```python
from build123d import *
from build123d.topology import SkipClean

# Parameters (mm, degrees)
SKETCH_1_W           = 51
SKETCH_1_H           = 30
EXTRUDE_5_DEPTH      = 7.5
SKETCH_4_W           = 31
SKETCH_4_H           = 30
EXTRUDE_6_DEPTH      = 20
SKETCH_6_W           = 5.5
SKETCH_6_H           = 10
EXTRUDE_9_DEPTH      = 3
SKETCH_10_W          = 5.5
SKETCH_10_H          = 10
EXTRUDE_10_DEPTH     = 3
SKETCH_13_R          = 10.95
CUT_EXTRUDE_1_DEPTH  = 3.55
CUT_EXTRUDE_2_DEPTH  = 10.3
CUT_EXTRUDE_3_DEPTH  = 33.666075675
CUT_EXTRUDE_5_DEPTH  = 41.391830857
CUT_EXTRUDE_7_DEPTH  = 57.797887285
EXTRUDE_12_DEPTH     = 31
CUT_EXTRUDE_13_DEPTH = 57.79788732
EXTRUDE_14_DEPTH     = 7.5
CUT_EXTRUDE_14_DEPTH = 41.391830988


with BuildPart() as part:
    # Эскиз1 → Бобышка-Вытянуть5 (new body)
    with BuildSketch(Plane.XY):
        Rectangle(SKETCH_1_W, SKETCH_1_H)
    extrude(amount=EXTRUDE_5_DEPTH)

    # Эскиз4 → Бобышка-Вытянуть6 (add)
    with BuildSketch(Plane(origin=(0, 0, 0), x_dir=(-1, 0, 0), z_dir=(0, 0, -1))):
        with Locations((10, 0)):
            Rectangle(SKETCH_4_W, SKETCH_4_H)
    extrude(amount=EXTRUDE_6_DEPTH)

    # Эскиз6 → Бобышка-Вытянуть9 (add)
    with BuildSketch(Plane(origin=(0, 0, 0), x_dir=(-1, 0, 0), z_dir=(0, 0, -1))):
        with Locations((-15.5, 10)):
            Rectangle(SKETCH_6_W, SKETCH_6_H)
        with Locations((-15.5, -10)):
            Rectangle(SKETCH_6_W, SKETCH_6_H)
    extrude(amount=EXTRUDE_9_DEPTH)

    # Эскиз10 → Бобышка-Вытянуть10 (add)
    with BuildSketch(Plane(origin=(5.5, 0, 0), x_dir=(0, 0, -1), z_dir=(1, 0, 0))):
        with Locations((10, 10)):
            Rectangle(SKETCH_10_W, SKETCH_10_H)
        with Locations((10, -10)):
            Rectangle(SKETCH_10_W, SKETCH_10_H)
    extrude(amount=EXTRUDE_10_DEPTH)

    # Эскиз13 → Вырез-Вытянуть1 (cut)
    with BuildSketch(Plane.XY.offset(7.5)):
        with Locations((-10, 0)):
            Circle(SKETCH_13_R)
    extrude(amount=-CUT_EXTRUDE_1_DEPTH, mode=Mode.SUBTRACT)

    # Эскиз14 → Вырез-Вытянуть2 (cut)
    with BuildSketch(Plane.XY.offset(3.95)):
        with BuildLine():
            ThreePointArc((-4.91, 0), (-6.400826484, 3.599173516), (-10, 5.09))
            Line((-10, 5.09), (-10, -5.09))
            ThreePointArc((-10, -5.09), (-6.400826484, -3.599173516), (-4.91, 0))
        make_face()
        with BuildLine():
            Line((-10, -5.09), (-10, 5.09))
            ThreePointArc((-10, 5.09), (-15.09, 0), (-10, -5.09))
        make_face()
    extrude(amount=-CUT_EXTRUDE_2_DEPTH, mode=Mode.SUBTRACT)

    # Эскиз15 → Вырез-Вытянуть3 (cut, through all)
    with BuildSketch(Plane.XY.offset(-6.35)):
        with BuildLine():
            ThreePointArc((-5.7, 0), (-6.959440841, 3.040559159), (-10, 4.3))
            Line((-10, 4.3), (-10, -4.3))
            ThreePointArc((-10, -4.3), (-6.959440841, -3.040559159), (-5.7, 0))
        make_face()
        with BuildLine():
            Line((-10, -4.3), (-10, 4.3))
            ThreePointArc((-10, 4.3), (-14.3, 0), (-10, -4.3))
        make_face()
    extrude(amount=-CUT_EXTRUDE_3_DEPTH, mode=Mode.SUBTRACT)

    # Эскиз16 → Вырез-Вытянуть5 (cut, through all)
    with BuildSketch(Plane.XY.offset(7.5)):
        with BuildLine():
            ThreePointArc((18.3, 0), (17.479898987, 1.979898987), (15.5, 2.8))
            Line((15.5, 2.8), (15.5, -2.8))
            ThreePointArc((15.5, -2.8), (17.479898987, -1.979898987), (18.3, 0))
        make_face()
        with BuildLine():
            Line((15.5, -2.8), (15.5, 2.8))
            ThreePointArc((15.5, 2.8), (12.7, 0), (15.5, -2.8))
        make_face()
    extrude(amount=-CUT_EXTRUDE_5_DEPTH, mode=Mode.SUBTRACT)

    # Эскиз17 → Вырез-Вытянуть7 (cut, through all)
    with SkipClean():  # the faces are left unmerged after this step: merging them gives an invalid solid
        with BuildSketch(Plane.ZY.offset(25.5)):
            with BuildLine():
                ThreePointArc((-12.6, 0), (-10, -2.6), (-7.4, 0))
                Line((-7.4, 0), (-12.6, 0))
            make_face()
            with BuildLine():
                Line((-12.6, 0), (-7.4, 0))
                ThreePointArc((-7.4, 0), (-10, 2.6), (-12.6, 0))
            make_face()
        extrude(amount=-CUT_EXTRUDE_7_DEPTH, mode=Mode.SUBTRACT)

    # Эскиз23 → Бобышка-Вытянуть12 (add)
    with SkipClean():  # the faces are left unmerged after this step: merging them gives an invalid solid
        with BuildSketch(Plane.ZY.offset(25.5)):
            with BuildLine():
                ThreePointArc((-12.6, 0), (-10, -2.6), (-7.4, 0))
                Line((-7.4, 0), (-12.6, 0))
            make_face()
            with BuildLine():
                Line((-12.6, 0), (-7.4, 0))
                ThreePointArc((-7.4, 0), (-10, 2.6), (-12.6, 0))
            make_face()
        extrude(amount=-EXTRUDE_12_DEPTH)

    # Эскиз24 → Вырез-Вытянуть13 (cut, through all)
    with BuildSketch(Plane.ZY.offset(25.5)):
        with BuildLine():
            ThreePointArc((-7.15, 0), (-10, 2.85), (-12.85, 0))
            Line((-12.85, 0), (-7.15, 0))
        make_face()
        with BuildLine():
            Line((-7.15, 0), (-12.85, 0))
            ThreePointArc((-12.85, 0), (-10, -2.85), (-7.15, 0))
        make_face()
    extrude(amount=-CUT_EXTRUDE_13_DEPTH, mode=Mode.SUBTRACT)

    # Эскиз27 → Бобышка-Вытянуть14 (add)
    with BuildSketch(Plane.XY.offset(7.5)):
        with BuildLine():
            ThreePointArc((15.5, 2.8), (12.7, 0), (15.5, -2.8))
            Line((15.5, -2.8), (15.5, 2.8))
        make_face()
        with BuildLine():
            Line((15.5, 2.8), (15.5, -2.8))
            ThreePointArc((15.5, -2.8), (17.479898987, -1.979898987), (18.3, 0))
            ThreePointArc((18.3, 0), (17.479898987, 1.979898987), (15.5, 2.8))
        make_face()
    extrude(amount=-EXTRUDE_14_DEPTH)

    # Эскиз28 → Вырез-Вытянуть14 (cut, through all)
    with BuildSketch(Plane.XY.offset(7.5)):
        with BuildLine():
            ThreePointArc((15.5, 2.85), (12.65, 0), (15.5, -2.85))
            Line((15.5, -2.85), (15.5, 2.85))
        make_face()
        with BuildLine():
            Line((15.5, 2.85), (15.5, -2.85))
            ThreePointArc((15.5, -2.85), (17.515254326, -2.015254326), (18.35, 0))
            ThreePointArc((18.35, 0), (17.515254326, 2.015254326), (15.5, 2.85))
        make_face()
    extrude(amount=-CUT_EXTRUDE_14_DEPTH, mode=Mode.SUBTRACT)


solid = part.part
```
Here's how the part is built. I have some questions about the finished solid (model axes, mm). A direction names the side the tool comes from. Coordinates: 2 decimals unless noted, no trailing zeros. Order: outer loops, then holes, each group sorted by start corner. A loop starts at its lowest first (then second) coordinate and runs counter-clockwise, first axis right, second up. Notation, with made-up numbers: (-26.5, 27) -> (25.5, 27) arc R6 ccw to (25.5, 34) -> close; hole circle Ø9 at (-36, -21.75). An arc over 180 degrees is marked (long way). Return JSON: item names as keys, results as strings.
1) If we section it at D-D on y = -12.5: List the corners of the cut face in (x, z) for me, plus the area to 3 significant figures.
Conclusion:
{"outline": "(-25.5, -20) -> (5.5, -20) -> (5.5, -12.75) -> (8.5, -12.75) -> (8.5, -7.25) -> (5.5, -7.25) -> (5.5, 0) -> (12.75, 0) -> (12.75, -3) -> (18.25, -3) -> (18.25, 0) -> (25.5, 0) -> (25.5, 7.5) -> (-25.5, 7.5) -> close", "area": "1,040 mm²"}
2) Thinking about a two-plate mould opening in X: for faces 1 (the flat face through (12.75, -10, -1)), 2 (the flat face through (7, 10, -12.75)), 3 (the flat face through (8.5, 10, -10)), which applies, +X half, -X half, draft (parallel to the pull), parting line (faces both ways), or undercut?
Conclusion:
{"face 1": "undercut", "face 2": "draft", "face 3": "+X half"}
3) If we section it at B-B on x = 6.5: List the corners of the cut face in (y, z) for me.
Conclusion:
{"outline": "(-15, -12.75) -> (-5, -12.75) -> (-5, -7.25) -> (-15, -7.25) -> close; (-15, 0) -> (15, 0) -> (15, 7.5) -> (-15, 7.5) -> close; (5, -12.75) -> (15, -12.75) -> (15, -7.25) -> (5, -7.25) -> close"}
4) I'm going to push flat-ended pins straight in: P1, Ø1.6, axis at y = 11.5, z = -10.5, coming from the +X side; P2, Ø17.5, axis at x = -10, y = 0, coming from the +Z side; P3, Ø4.5, axis at x = 16, y = 11, coming from the -Z side; P4, Ø1, axis at x = 8, z = -14.5, coming from the +Y side. Where does each tip first touch, or does it pass through?
Conclusion:
{"P1": "stops at x = 8.5", "P2": "stops at z = 3.95", "P3": "stops at z = -3", "P4": "passes through"}
5) If we section it at C-C on y = -2.25: State how many separate pieces and enclosed holes the cut face has, plus the area to 3 significant figures.
Conclusion:
{"separate pieces": "5", "enclosed holes": "0", "area": "623 mm²"}
6) If we section it at A-A on z = -10: List the corners of the cut face in (x, y) for me, plus the area to 3 significant figures.
Conclusion:
{"outline": "(-25.5, -15) -> (8.5, -15) -> (8.5, -5) -> (5.5, -5) -> (5.5, -2.85) -> (-6.78, -2.85) arc R4.3 cw to (-13.22, -2.85) -> (-25.5, -2.85) -> close; (-25.5, 2.85) -> (-13.22, 2.85) arc R4.3 cw to (-6.78, 2.85) -> (5.5, 2.85) -> (5.5, 5) -> (8.5, 5) -> (8.5, 15) -> (-25.5, 15) -> close", "area": "800 mm²"}
7) If I drill on probe 1 along Y at (x, z) = (0.25, -10); probe 2 along Z at (x, y) = (2.5, 0); probe 3 along Y at (x, z) = (-10, 4.7), over which ranges is the centre line in solid material (lowest first)?
Conclusion:
{"probe 1": "y = -15 to -2.85, 2.85 to 15", "probe 2": "z = -20 to -12.85, -7.15 to 7.5", "probe 3": "y = -15 to -10.95, 10.95 to 15"}
8) On a 3-axis mill with a long thin cutter (end or side, diameter ignored), from which of +Z, -Z, +X, -X, +Y, -Y can I reach the whole of each face in a straight line? I mean faces 4 (the flat face through (8.5, -10, -10)), 5 (the flat face through (7, 5, -10)), 6 (the flat face through (12.75, 10, -1)), 7 (the flat face through (7, -10, -7.25)). Say none if no direction works.
Conclusion:
{"face 4": "-Z, +X, +Y, -Y", "face 5": "-Z, +X", "face 6": "-Z, +Y, -Y", "face 7": "+X, +Y, -Y"}
